Verification items for this drawing (mm, ordinates from the low corner). A direction names the side the tool comes from. Give positions to 0.01 mm unless a question says otherwise; leave off trailing zeros. Write each loop counter-clockwise with the first axis right and the second up, starting at its lowest first coordinate (ties: lowest second). Pieces come first, ordered by that corner, then holes. Notation, with made-up numbers: (-23.75, 84) -> (-12.75, 84) arc R16 cw to (-12.75, 89) -> close; hole circle Ø6 at (79.5, 48). An arc over 180 degrees is marked (long way). Write item = value, one per line.
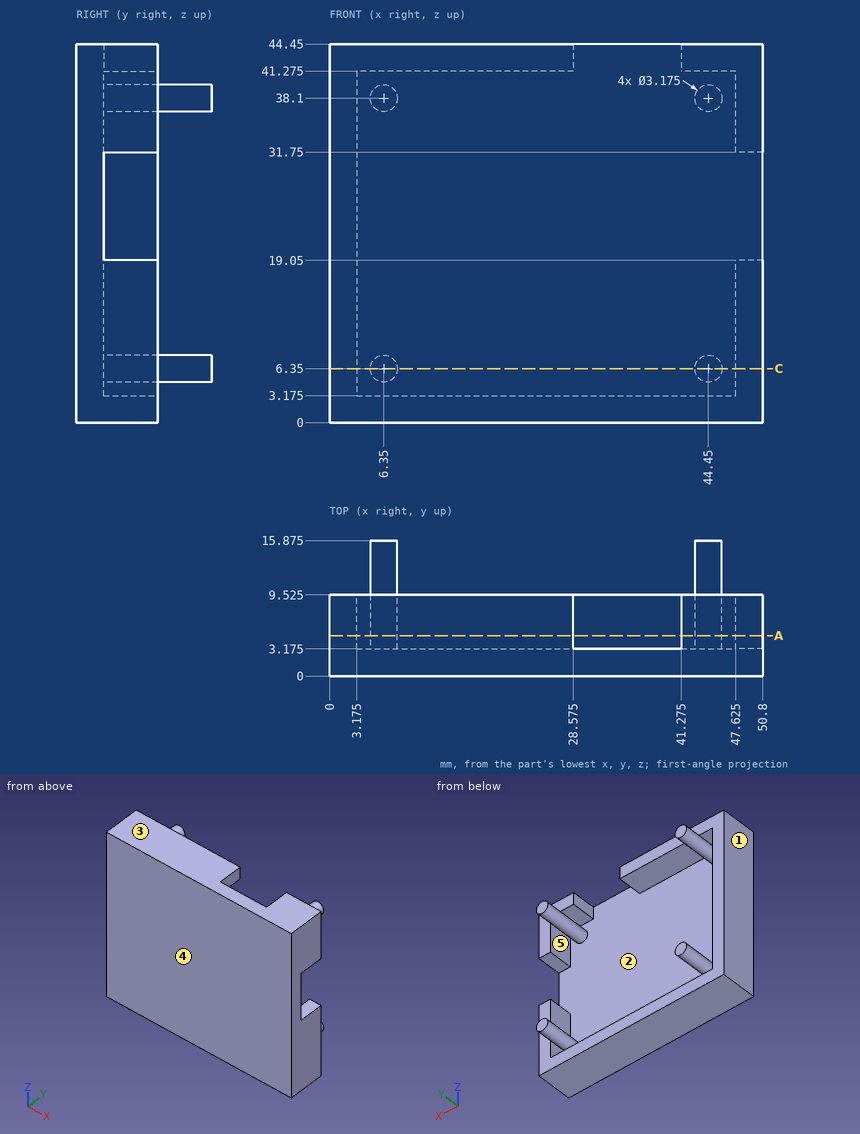
Item 1: Sectioned sample at A-A on y = 4.75. Give the number of separate pieces and of enclosed holes in the cut face, then the cut area to 3 significant figures.
Response values:
separate_pieces = 6
enclosed_holes = 0
area = 516 mm^2
Item 2: Material ranges on line 1 (Z direction, x = 11.5, y = 4.25) (3 decimals); line 2 (X direction, y = 6, z = 9) (3 decimals); line 3 (Y direction, x = 38, z = 38.5) (3 decimals), recorded low to high.
Response values:
line_1 = 0 to 3.175, 41.275 to 44.45
line_2 = 0 to 3.175, 47.625 to 50.8
line_3 = 0 to 3.175
Item 3: Mould release check, pull along Z, two halves, no side actions. Record for the marked faces 1, 2 and 3: +Z half, -Z half, draft (parallel to the pull), parting line (faces both ways), or undercut.
Response values:
face_1 = draft
face_2 = undercut
face_3 = +Z half
Item 4: Sectioned sample at C-C on z = 6.35. Record the cut outline in (x, y) (1 decimal), then the cut area to 3 significant figures.
Response values:
outline = (0, 0) -> (50.8, 0) -> (50.8, 9.5) -> (47.6, 9.5) -> (47.6, 3.2) -> (46, 3.2) -> (46, 15.9) -> (42.9, 15.9) -> (42.9, 3.2) -> (7.9, 3.2) -> (7.9, 15.9) -> (4.8, 15.9) -> (4.8, 3.2) -> (3.2, 3.2) -> (3.2, 9.5) -> (0, 9.5) -> close
area = 282 mm^2
Item 5: Set-up check for the marked faces 4 and 5: record each of +Z, -Z, +X, -X, +Y, -Y from which the full face is reachable in a straight line by a thin tool's end or side.
Response values:
face_4 = +Z, -Z, +X, -X, -Y
face_5 = +Y
Item 6: Go/stop test with flat-tipped pins: P1, Ø1.5, axis at x = 37.5, y = 7.5, coming from the +Z side (3 decimals); P2, Ø2, axis at x = 12.5, z = 34.5, coming from the +Y side (3 decimals); P3, Ø8, axis at x = 6.5, z = 19.5, coming from the +Y side (3 decimals). Record where each tip stops, or that it passes through.
Response values:
P1 = 3.175
P2 = 3.175
P3 = 9.525
